Work out the finished part from the listing and answer in its coordinate system (mm). A direction names the side the tool comes from. Give positions to 0.01 mm unless a question says otherwise; leave off trailing zeros. Order: outer loops, then holes, each group sorted by start corner. A loop starts at its lowest first (then second) coordinate and runs counter-clockwise, first axis right, second up.
```python
from build123d import *

# Parameters (mm, degrees)
CHAMFER_1_SIZE      = 1
CUT_EXTRUDE_START   = -3
SKETCH_2_R          = 5
SKETCH_2_R_2        = 4.8
CUT_EXTRUDE_1_DEPTH = 1.1


with BuildPart() as part:
    # 草图1 → 旋转1 (revolve)
    with BuildSketch(Plane.XY, mode=Mode.PRIVATE) as revolve_1_sk:
        Polygon((0, 54), (5, 54), (5, 30), (5, -30), (5, -54), (0, -54), align=None)
    revolve(revolve_1_sk.sketch.rotate(Axis((0, 54, 0), (0, -1, 0)), 180), axis=Axis((0, 54, 0), (0, -1, 0)))

    # 倒角1
    chamfer_1_edges = [part.edges().sort_by_distance(p)[0] for p in [
        (5, -54, 0),
        (5, 54, 0),
    ]]
    chamfer(chamfer_1_edges, length=CHAMFER_1_SIZE)

    # 草图2 → 切除-拉伸1 (cut)
    with BuildSketch(Plane(origin=(0, 54, 0), x_dir=(1, 0, 0), z_dir=(0, 1, 0)).offset(CUT_EXTRUDE_START)):
        with Locations(Location((0, 0, 0), (0, 0, 180))):
            Circle(SKETCH_2_R)
        with Locations(Location((0, 0, 0), (0, 0, 180))):
            Circle(SKETCH_2_R_2, mode=Mode.SUBTRACT)
    cut_extrude_1 = extrude(amount=CUT_EXTRUDE_1_DEPTH, mode=Mode.SUBTRACT)

    # 镜向1: 切除-拉伸1 across plane
    add(cut_extrude_1.mirror(Plane.ZX), mode=Mode.SUBTRACT)


solid = part.part
```
1. The mould has two halves that part along Y. Classify faces 1 (the face through (4.995, 52.556, -0.22)), 2 (the face through (-2.58, -51.54, 4.05)), 3 (the face through (0, 54, 0)): pulls with the +Y half, pulls with the -Y half, needs draft (parallel to the pull), parting line crosses it, or undercut.
Findings below:
face 1: needs draft
face 2: undercut
face 3: pulls with the +Y half
2. Which of the six approach directions +Z, -Z, +X, -X, +Y, -Y give full straight-line access (tool end or side, diameter ignored) to faces 4 (the face through (-2.58, 51.54, 4.05)), 5 (the face through (0, -54, 0))?
Findings below:
face 4: none
face 5: +Z, -Z, +X, -X, -Y
3. The part is cut by section A-A (y = -5.5). Write down the section's boundary in (x, z), then the cut area to 3 significant figures.
Findings below:
outline: circle Ø10 at (0, 0)
area: 78.5 mm2
4. Straight lines are drawn through the part: probe 1 along X at (y, z) = (41, 1.25); probe 2 along Z at (x, y) = (-2.5, 5.5); probe 3 along Z at (x, y) = (-1, -16). For each, find the intervals that lie inside material, in ascending order.
Findings below:
probe 1: x = -4.84 to 4.84
probe 2: z = -4.33 to 4.33
probe 3: z = -4.9 to 4.9
5. Given P1, Ø4, axis at x = 3, y = -1.5, coming from the -Z side, flat-ended and moving along its own axis, determine where the tip first touches the part or whether it passes through.
Findings below:
P1: stops at z = -4.9
